Source: CAD feature listing. Evaluate the final solid. Frame: model axes, mm. A direction names the side the tool comes from. Give positions to 0.01 mm unless a question says otherwise; leave off trailing zeros. Loops run counter-clockwise (first coordinate to the right, second up) from the corner with the lowest first, then second, coordinate; pieces in that order, holes last. Notation, with made-up numbers: (-24.75, 21) -> (-4.75, 21) arc R7 ccw to (-4.75, 25) -> close; hole circle Ø6 at (47, 45.25). An arc over 180 degrees is marked (long way). Return JSON: item names as keys, results as strings. Group by question number.
(1) Cut plane D-D on y = 3.5. Return loops of the section in (x, z) (3 decimals), then the cut area to 3 significant figures.
(2) Access query for faces 4 (the face through (3, -1, -5.4)), 5 (the face through (2.725, 4.5, 6)), 6 (the face through (2, 2.53, 4)). Directions: +Z, -Z, +X, -X, +Y, -Y. A direction counts if a zero-diameter tool reaches every point of the face in a straight line with its end or side. Return the directions, or none.
(3) Draft query along Y for faces 1 (the face through (2, 4.5, 7.09)), 2 (the face through (3.33, 5.001, 4.924)), 3 (the face through (1.375, 3, 4)). Return one class per face: released by +Y, released by -Y, zero draft, split by the parting line, or undercut.
(4) Ray query, line 1 (Y direction, x = 4, z = 4.5); line 2 (Y direction, x = 1.5, z = 0); line 3 (Z direction, x = 3.25, y = -2.5). Return the intervals inside material, ascending. Write a range as from..to.
(5) Pin query (flat end, axial travel): pin 1 (1 mm diameter, centred on x = 2, z = -3.5, fed in from -Y); pin 2 (2 mm diameter, centred on x = 2.5, y = -2, fed in from +Z); pin 3 (0.6 mm diameter, centred on y = 4.5, z = 6, fed in from -X) (3 decimals); pin 4 (0.9 mm diameter, centred on y = 4.5, z = 6, fed in from +X) (3 decimals). Return the tip coordinate at first contact, or that it passes through.
(6) Cut plane C-C on y = -5.75. Return loops of the section in (x, z), then the cut area to 3 significant figures.
(7) Cut plane B-B on x = 2.05. Return loops of the section in (y, z).
(8) Cut plane A-A on z = 3.56. Return loops of the section in (x, y) (3 decimals).
```python
from build123d import *

# Parameters (mm, degrees)
SKETCH_1_W          = 10.8
SKETCH_1_H          = 10.3
EXTRUDE_1_DEPTH     = 6.64
CHAMFER_1_SIZE      = 2
SKETCH_2_R          = 0.3
EXTRUDE_2_DEPTH     = 3.2
FILLET_1_R          = 1
SKETCH_3_W          = 1.35
SKETCH_3_H          = 2.620478626
CUT_EXTRUDE_1_DEPTH = 2
SKETCH_4_W          = 3.89
SKETCH_4_H          = 2.620478626
CUT_EXTRUDE_2_DEPTH = 0.1
SKETCH_5_W          = 1.35
SKETCH_5_H          = 1
EXTRUDE_3_DEPTH     = 3.69
CHAMFER_2_SIZE      = 0.1


with BuildPart() as part:
    # Эскиз1 → Вытянуть1 (new body)
    with BuildSketch(Plane(origin=(0, 0, 0), x_dir=(0, 0, -1), z_dir=(1, 0, 0))):
        Rectangle(SKETCH_1_W, SKETCH_1_H)
    extrude(amount=EXTRUDE_1_DEPTH)

    # Фаска1
    chamfer_1_edges = [part.edges().sort_by_distance(p)[0] for p in [
        (3.32, 5.15, -5.4),
    ]]
    chamfer(chamfer_1_edges, length=CHAMFER_1_SIZE)

    # Эскиз2 → Вытянуть2 (add)
    with BuildSketch(Plane.XZ.offset(5.15)):
        with Locations(Location((2.05, 3.56, 0), (0, 0, 90))):
            Circle(SKETCH_2_R)
        with Locations(Location((4.59, 3.56, 0), (0, 0, 90))):
            Circle(SKETCH_2_R)
        with Locations(Location((2.05, -4.06, 0), (0, 0, 90))):
            Circle(SKETCH_2_R)
        with Locations(Location((4.59, -4.06, 0), (0, 0, 90))):
            Circle(SKETCH_2_R)
    extrude(amount=EXTRUDE_2_DEPTH)

    # Скругление1
    fillet_1_edges = [part.edges().sort_by_distance(p)[0] for p in [
        (3.32, 5.15, 5.4),
    ]]
    fillet(fillet_1_edges, radius=FILLET_1_R)

    # Эскиз3 → Вырез-Вытянуть1 (cut)
    with BuildSketch(Plane.XY.offset(5.4)):
        with Locations((2.05, 3.839760687)):
            Rectangle(SKETCH_3_W, SKETCH_3_H)
        with Locations((4.59, 3.839760687)):
            Rectangle(SKETCH_3_W, SKETCH_3_H)
    extrude(amount=-CUT_EXTRUDE_1_DEPTH, mode=Mode.SUBTRACT)

    # Эскиз4 → Вырез-Вытянуть2 (cut)
    with BuildSketch(Plane.XY.offset(5.4)):
        with Locations((3.32, 3.839760687)):
            Rectangle(SKETCH_4_W, SKETCH_4_H)
    extrude(amount=-CUT_EXTRUDE_2_DEPTH, mode=Mode.SUBTRACT)

    # Эскиз5 → Вытянуть3 (add)
    with BuildSketch(Plane.XY.offset(3.4)):
        with Locations((2.05, 4.528321525)):
            Rectangle(SKETCH_5_W, SKETCH_5_H)
        with Locations((4.59, 4.528321525)):
            Rectangle(SKETCH_5_W, SKETCH_5_H)
    extrude(amount=EXTRUDE_3_DEPTH)

    # Фаска2
    chamfer_2_edges = [part.edges().sort_by_distance(p)[0] for p in [
        (1.375, 5.028321525, 5.984035196),
        (1.375, 4.028321525, 6.245),
        (2.725, 4.028321525, 6.195),
        (2.725, 5.028321525, 5.984035196),
        (1.375, 4.528321525, 7.09),
        (2.05, 4.028321525, 7.09),
        (2.725, 4.528321525, 7.09),
        (2.05, 5.028321525, 7.09),
        (5.265, 4.028321525, 6.245),
        (3.915, 5.028321525, 5.984035196),
        (3.915, 4.028321525, 6.195),
        (5.265, 5.028321525, 5.984035196),
        (3.915, 4.528321525, 7.09),
        (4.59, 4.028321525, 7.09),
        (5.265, 4.528321525, 7.09),
        (4.59, 5.028321525, 7.09),
    ]]
    chamfer(chamfer_2_edges, length=CHAMFER_2_SIZE)


solid = part.part
```
Answers:
{
 "1": {"outline": "(0, -5.05) -> (6.64, -5.05) -> (6.64, 5.4) -> (5.265, 5.4) -> (5.265, 3.4) -> (3.915, 3.4) -> (3.915, 5.3) -> (2.725, 5.3) -> (2.725, 3.4) -> (1.375, 3.4) -> (1.375, 5.4) -> (0, 5.4) -> close", "area": "63.9 mm²"},
 "2": {"face 4": "-Z, +X, -X, +Y, -Y", "face 5": "+Z, +Y", "face 6": "+Z"},
 "3": {"face 1": "zero draft", "face 2": "released by +Y", "face 3": "undercut"},
 "4": {"line 1": "-5.15..2.53, 4.03..5.03", "line 2": "-5.15..5.15", "line 3": "-5.4..5.4"},
 "5": {"pin 1": "y = -8.35", "pin 2": "z = 5.4", "pin 3": "x = 1.375", "pin 4": "x = 5.265"},
 "6": {"outline": "circle Ø0.6 at (2.05, -4.06); circle Ø0.6 at (2.05, 3.56); circle Ø0.6 at (4.59, -4.06); circle Ø0.6 at (4.59, 3.56)", "area": "1.13 mm²"},
 "7": {"outline": "(-8.35, -4.36) -> (-5.15, -4.36) -> (-5.15, -5.4) -> (3.15, -5.4) -> (5.15, -3.4) -> (5.15, 3.4) -> (5.03, 3.4) -> (5.03, 6.99) -> (4.93, 7.09) -> (4.13, 7.09) -> (4.03, 6.99) -> (4.03, 3.4) -> (2.53, 3.4) -> (2.53, 5.4) -> (-5.15, 5.4) -> (-5.15, 3.86) -> (-8.35, 3.86) -> (-8.35, 3.26) -> (-5.15, 3.26) -> (-5.15, -3.76) -> (-8.35, -3.76) -> close"},
 "8": {"outline": "(0, -5.15) -> (1.75, -5.15) -> (1.75, -8.35) -> (2.35, -8.35) -> (2.35, -5.15) -> (4.29, -5.15) -> (4.29, -8.35) -> (4.89, -8.35) -> (4.89, -5.15) -> (6.64, -5.15) -> (6.64, 5.15) -> (5.265, 5.15) -> (5.265, 5.028) -> (3.915, 5.028) -> (3.915, 5.15) -> (2.725, 5.15) -> (2.725, 5.028) -> (1.375, 5.028) -> (1.375, 5.15) -> (0, 5.15) -> close; hole (1.375, 2.53) -> (2.725, 2.53) -> (2.725, 4.028) -> (1.375, 4.028) -> close; hole (3.915, 2.53) -> (5.265, 2.53) -> (5.265, 4.028) -> (3.915, 4.028) -> close"}
}
